Design review of the part shown in the three views and the two pictorial views. Dimensions are in mm from the part's minimum x, y and z. Round coordinates to 2 decimals unless told otherwise and drop trailing zeros. Loops run counter-clockwise (first coordinate to the right, second up) from the corner with the lowest first, then second, coordinate; pieces in that order, holes last.
1. Consider section B-B on y = 69.5. State the section outline as (x, z) points.
2. Consider section A-A on x = 67.5. State the section outline as (y, z) points, then the cut area to 3 significant figures.
3. Consider section C-C on z = 2.8. State the section outline as (x, y) points.
4. Clearance check with flat-ended pins moving along their axes: pin 1 Ø2.5 at (y, z) = (53, 3.5) entering from -X; pin 2 Ø2.5 at (x, z) = (35.5, 3) entering from -Y; pin 3 Ø3 at (x, y) = (67.5, 63.82) entering from +Z; pin 4 Ø2.5 at (y, z) = (49, 3.5) entering from +X. State where each tip first meets the part, or that it passes through.
5. To check wall thickness, follow line 1 along X through (y, z) = (63.5, 1.1); line 2 along Y through (x, z) = (27.5, 1.75); line 3 along X through (y, z) = (35, 0.9). State the ranges of each line that lie inside material, in increasing order.
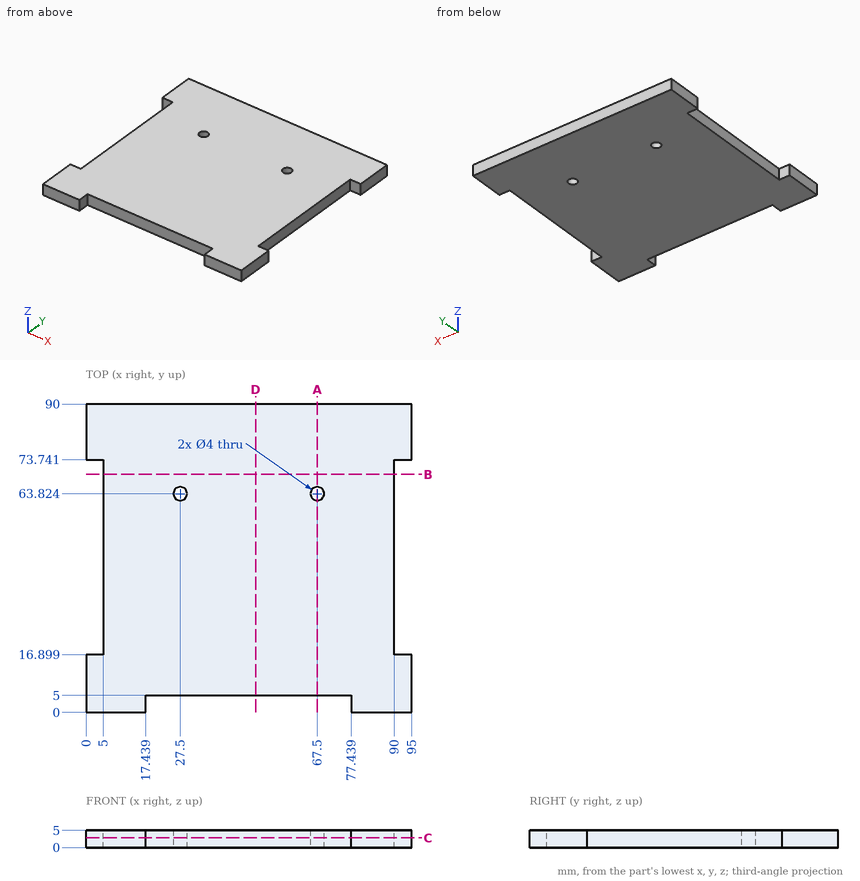
Resolved:
1. outline: (5, 0) - (90, 0) - (90, 5) - (5, 5) - close
2. outline: (5, 0) - (61.82, 0) - (61.82, 5) - (5, 5) - close; (65.82, 0) - (90, 0) - (90, 5) - (65.82, 5) - close
2. area: 405 mm2
3. outline: (0, 0) - (17.44, 0) - (17.44, 5) - (77.44, 5) - (77.44, 0) - (95, 0) - (95, 16.9) - (90, 16.9) - (90, 73.74) - (95, 73.74) - (95, 90) - (0, 90) - (0, 73.74) - (5, 73.74) - (5, 16.9) - (0, 16.9) - close; hole circle Ø4 at (27.5, 63.82); hole circle Ø4 at (67.5, 63.82)
4. pin 1: stops at x = 5
4. pin 2: stops at y = 5
4. pin 3: passes through
4. pin 4: stops at x = 90
5. line 1: x = 5 to 25.53, 29.47 to 65.53, 69.47 to 90
5. line 2: y = 5 to 61.82, 65.82 to 90
5. line 3: x = 5 to 90
